```python
from build123d import *

# Parameters (mm, degrees)
F0_W     = 19.05
F0_H     = 16.51
F0_W_2   = 1.25
F0_H_2   = 1.74
F0_R     = 1
F1_DEPTH = 1.8
F2_DEPTH = 2.2
F3_R     = 2.54


with BuildPart() as f1:
    # F0 (on Front) → F1 (new body)
    with BuildSketch(Plane.XZ):
        Rectangle(F0_W, F0_H)
        with Locations((0, -1.397)):
            Rectangle(F0_W_2, F0_H_2, mode=Mode.SUBTRACT)
        with Locations((-6.985, 5.715)):
            Circle(F0_R, mode=Mode.SUBTRACT)
        with Locations((6.985, 5.715)):
            Circle(F0_R, mode=Mode.SUBTRACT)
    extrude(amount=F1_DEPTH)

    # F0 (on Front) → F2 (join)
    with BuildSketch(Plane.XZ):
        with Locations((0, -1.397)):
            Rectangle(F0_W_2, F0_H_2)
    extrude(amount=F2_DEPTH)

    # F3
    f3_edges = [f1.edges().sort_by_distance(p)[0] for p in [
        (-9.525, -0.9, 8.255),
        (9.525, -0.9, 8.255),
        (9.525, -0.9, -8.255),
        (-9.525, -0.9, -8.255),
    ]]
    fillet(f3_edges, radius=F3_R)


solid = f1.part
```
Model file for the job. Use its own axes, mm. Coordinates: 2 decimals unless noted, no trailing zeros. Loops run counter-clockwise (first coordinate to the right, second up) from the corner with the lowest first, then second, coordinate; pieces in that order, holes last. Notation, with made-up numbers: (37.25, 74) - (43.25, 74) arc R22 ccw to (43.25, 97) - close; hole circle Ø1 at (73, 76.5). An arc over 180 degrees is marked (long way). Answer as a JSON object with one key per item and string values. Group by question number.
(1) Cut at C-C (x = 8.25). Give the cut face in (y, z).
(2) Cut at D-D (z = 3.5). Give the cut face in (x, y) (3 decimals).
(3) Cut at B-B (y = -1.55). Give the cut face in (x, z) (3 decimals), then the cut area to 3 significant figures.
(4) Two-plate mould, pull along Z, no slides. Class faces 1 (the face through (5.986, -0.887, 5.759)), 2 (the face through (8.76, -0.91, 7.53)), 3 (the face through (-8.8, -0.91, -7.49)): released by +Z, released by -Z, zero draft, split by the parting line, or undercut.
(5) Flat gauge pins, fed straight in: pin 1 (5 mm diameter, centred on x = -1.5, z = -5, fed in from -Y); pin 2 (1.5 mm diameter, centred on x = -6, z = 4, fed in from +Y). Where does each tip first touch, or does it go through?
(6) Cut at A-A (z = 6). Give the cut face in (x, y).
(7) Probe line 1 along X through (y, z) = (-1.2, 5.25) (3 decimals); line 2 along Y through (x, z) = (-6.25, 4.25); line 3 along X through (y, z) = (-0.65, 6). List the from-to ranges inside material, lowest first.
Geometry says:
{
 "1": {"outline": "(-1.8, -7.92) - (0, -7.92) - (0, 7.92) - (-1.8, 7.92) - close"},
 "2": {"outline": "(-9.525, -1.8) - (9.525, -1.8) - (9.525, 0) - (-9.525, 0) - close"},
 "3": {"outline": "(-9.525, -5.715) arc R2.54 ccw to (-6.985, -8.255) - (6.985, -8.255) arc R2.54 ccw to (9.525, -5.715) - (9.525, 5.715) arc R2.54 ccw to (6.985, 8.255) - (-6.985, 8.255) arc R2.54 ccw to (-9.525, 5.715) - close; hole circle Ø2 at (-6.985, 5.715); hole circle Ø2 at (6.985, 5.715)", "area": "303 mm^2"},
 "4": {"face 1": "undercut", "face 2": "released by +Z", "face 3": "released by -Z"},
 "5": {"pin 1": "stops at y = -1.8", "pin 2": "stops at y = 0"},
 "6": {"outline": "(-9.51, -1.8) - (-7.94, -1.8) - (-7.94, 0) - (-9.51, 0) - close; (-6.03, -1.8) - (6.03, -1.8) - (6.03, 0) - (-6.03, 0) - close; (7.94, -1.8) - (9.51, -1.8) - (9.51, 0) - (7.94, 0) - close"},
 "7": {"line 1": "x = -9.525 to -7.87, -6.1 to 6.1, 7.87 to 9.525", "line 2": "y = -1.8 to 0", "line 3": "x = -9.51 to -7.94, -6.03 to 6.03, 7.94 to 9.51"}
}
